```python
from build123d import *

# Parameters (mm, degrees)
CROQUIS1_R              = 8
SALIENTE_EXTRUIR1_DEPTH = 14.5
CROQUIS2_R              = 1
CROQUIS2_R_2            = 1.51
CORTAR_EXTRUIR1_DEPTH   = 5
SALIENTE_EXTRUIR2_START = 2
CROQUIS3_R              = 3
CROQUIS3_R_2            = 1.51
SALIENTE_EXTRUIR2_DEPTH = 2
CROQUIS4_R              = 1.5
SALIENTE_EXTRUIR3_DEPTH = 18


with BuildPart() as part:
    # Croquis1 → Saliente-Extruir1 (new body)
    with BuildSketch(Plane(origin=(0, 0, 0), x_dir=(1, 0, 0), z_dir=(0, 1, 0))):
        with Locations(Location((0, 0, 0), (0, 0, 90))):
            Circle(CROQUIS1_R)
    extrude(amount=SALIENTE_EXTRUIR1_DEPTH)

    # Croquis2 → Cortar-Extruir1 (cut)
    with BuildSketch(Plane(origin=(0, 14.5, 0), x_dir=(1, 0, 0), z_dir=(0, 1, 0))):
        with Locations(Location((6, 0, 0), (0, 0, 270))):
            Circle(CROQUIS2_R)
        with Locations(Location((-6, 0, 0), (0, 0, 270))):
            Circle(CROQUIS2_R)
        with Locations(Location((0, 0, 0), (0, 0, 270))):
            Circle(CROQUIS2_R_2)
    extrude(amount=-CORTAR_EXTRUIR1_DEPTH, mode=Mode.SUBTRACT)

    # Croquis3 → Saliente-Extruir2 (add)
    with BuildSketch(Plane(origin=(0, 14.5, 0), x_dir=(1, 0, 0), z_dir=(0, 1, 0)).offset(SALIENTE_EXTRUIR2_START)):
        with Locations(Location((0, 0, 0), (0, 0, 270))):
            Circle(CROQUIS3_R)
        with Locations(Location((0, 0, 0), (0, 0, 270))):
            Circle(CROQUIS3_R_2, mode=Mode.SUBTRACT)
    extrude(amount=-SALIENTE_EXTRUIR2_DEPTH)

    # Croquis4 → Saliente-Extruir3 (add)
    with BuildSketch(Plane(origin=(0, 9.5, 0), x_dir=(1, 0, 0), z_dir=(0, 1, 0))):
        with Locations(Location((0, 0, 0), (0, 0, 270))):
            Circle(CROQUIS4_R)
    extrude(amount=SALIENTE_EXTRUIR3_DEPTH)


solid = part.part
```
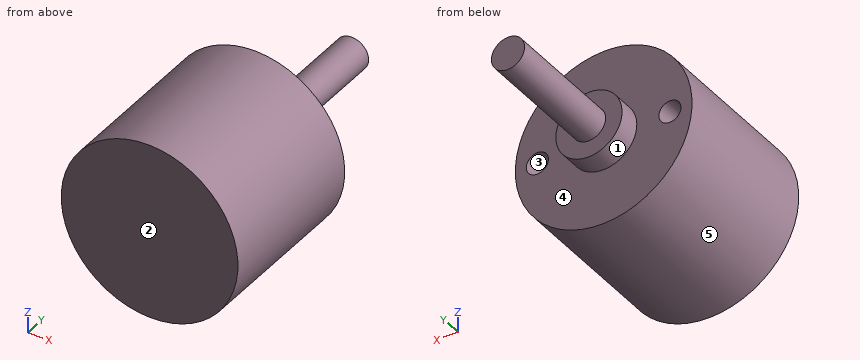
Here's how the part is built. I have some questions about the finished solid (model axes, mm). Face numbers are marked on the shaded views. A direction names the side the tool comes from. Give positions to 0.01 mm unless a question says otherwise; leave off trailing zeros. Order: outer loops, then holes, each group sorted by start corner. A loop starts at its lowest first (then second) coordinate and runs counter-clockwise, first axis right, second up. Notation, with made-up numbers: (-6.5, 34.25) - (14.5, 34.25) arc R18 ccw to (14.5, 69.25) - close; hole circle Ø2 at (38.5, 53.5). An arc over 180 degrees is marked (long way). Answer as a JSON object with one key per item and string values. Group by question number.
Item 1: If we section it at A-A on y = 13.75: Please give me the cut outline in (x, z), and give its area (3 significant figures).
Item 2: If we section it at D-D on y = 1.5: Please give me the cut outline in (x, z).
Item 3: Please list where these lines run through material, in increasing order: probe 1 along Y at (x, z) = (-4, 5); probe 2 along Y at (x, z) = (1.75, -2.25); probe 3 along X at (y, z) = (11.75, 1.75).
Item 4: Which directions (+Z, -Z, +X, -X, +Y, -Y) give clear straight access to the entire face, cutting with the end or side of a thin tool? Please do the marked faces 4 and 5.
Item 5: For P1, Ø2.5, axis at x = -6, z = 0, coming from the +Y side; P2, Ø6, axis at x = -3.5, y = 12.5, coming from the -Z side; P3, Ø0.6, axis at x = 6.5, z = 0, coming from the +Y side; P4, Ø3, axis at y = 22.5, z = -4, coming from the +X side, each with a flat end and sliding along its axis, tell me the tip position at first contact or that it passes through.
Item 6: If we mould it in two halves opening along X, with no side actions, what happens to the marked faces 1, 2 and 3? For each: pulls with the +X half, pulls with the -X half, needs draft (parallel to the pull), parting line crosses it, or undercut.
Result set:
{
 "1": {"outline": "circle Ø16 at (0, 0); circle Ø3 at (0, 0); hole circle Ø2 at (-6, 0); hole circle Ø3.02 at (0, 0); hole circle Ø2 at (6, 0)", "area": "195 mm²"},
 "2": {"outline": "circle Ø16 at (0, 0)"},
 "3": {"probe 1": "0 to 14.5", "probe 2": "0 to 16.5", "probe 3": "-7.81 to 7.81"},
 "4": {"face 4": "+Y", "face 5": "+Y, -Y"},
 "5": {"P1": "y = 14.5", "P2": "z = -7.98", "P3": "y = 9.5", "P4": "through"},
 "6": {"face 1": "parting line crosses it", "face 2": "needs draft", "face 3": "undercut"}
}
